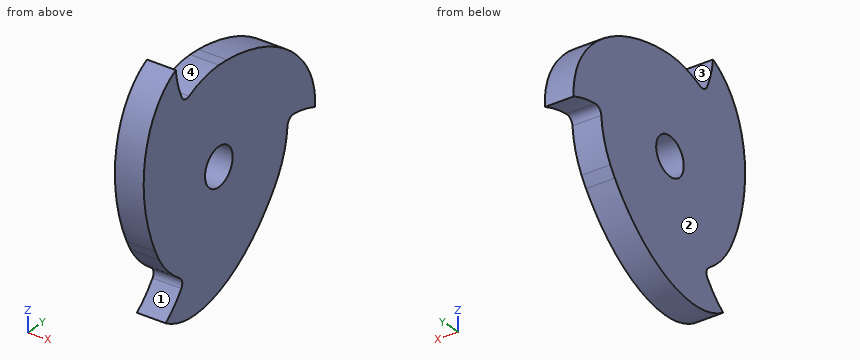
from build123d import *

# Parameters (mm, degrees)
SKETCH1_R           = 6.35
BOSS_EXTRUDE3_DEPTH = 9.525
FILLET3_R           = 2.54


with BuildPart() as part:
    # Sketch1 → Boss-Extrude3 (new body)
    # profile 1 of 4: a face of its own
    with BuildSketch(Plane(origin=(0, 0, 0), x_dir=(0, 0, -1), z_dir=(1, 0, 0))):
        with BuildLine():
            ThreePointArc((-31.520099492, 3.813899322), (-21.059097755, 23.760827043), (0, 31.75))
            ThreePointArc((0, 31.75), (0.675988504, 38.199887052), (2.67457554, 44.369461859))
            add(Edge.make_bspline(
                [(2.67457554, 44.369461859), (-27.656863026, 46.197830298), (-31.520099492, 3.813899322)],
                knots=[3.141592654, 3.141592654, 3.141592654, 4.660979846, 4.660979846, 4.660979846], degree=2, weights=[1, 0.709776495, 0.966045781]))
        make_face()
    # profile 2 of 4: a face of its own
    with BuildSketch(Plane(origin=(0, 0, 0), x_dir=(0, 0, -1), z_dir=(1, 0, 0))):
        with BuildLine():
            add(Edge.make_bspline(
                [(19.062983446, 25.390257228), (17.50131988, 26.492217898), (15.875, 27.49630657)],
                knots=[1.519387193, 1.519387193, 1.519387193, 1.613788447, 1.613788447, 1.613788447], degree=2, weights=[0.966045781, 0.981968084, 1]))
            ThreePointArc((15.875, 27.49630657), (8.217504682, 30.668144985), (0, 31.75))
            ThreePointArc((0, 31.75), (-21.059097755, 23.760827043), (-31.520099492, 3.813899322))
            add(Edge.make_bspline(
                [(-31.520099492, 3.813899322), (-31.693593642, 1.910478667), (-31.75, 0)],
                knots=[4.660979846, 4.660979846, 4.660979846, 4.7553811, 4.7553811, 4.7553811], degree=2, weights=[0.966045781, 0.981968084, 1]))
            ThreePointArc((-31.75, 0), (-30.668144985, -8.217504682), (-27.49630657, -15.875))
            ThreePointArc((-27.49630657, -15.875), (-10.047930956, -30.118127158), (12.457116045, -29.204156551))
            add(Edge.make_bspline(
                [(12.457116045, -29.204156551), (14.192273762, -28.402696564), (15.875, -27.49630657)],
                knots=[1.519387193, 1.519387193, 1.519387193, 1.613788447, 1.613788447, 1.613788447], degree=2, weights=[0.966045781, 0.981968084, 1]))
            ThreePointArc((15.875, -27.49630657), (22.450640303, -22.450640303), (27.49630657, -15.875))
            ThreePointArc((27.49630657, -15.875), (30.668144985, -8.217504682), (31.75, 0))
            ThreePointArc((31.75, 0), (28.401692066, 14.191771834), (19.062983446, 25.390257228))
        make_face()
        with Locations(Location((0, 0, 0), (0, 0, 180))):
            Circle(SKETCH1_R, mode=Mode.SUBTRACT)
    # profile 3 of 4: a face of its own
    with BuildSketch(Plane(origin=(0, 0, 0), x_dir=(0, 0, -1), z_dir=(1, 0, 0))):
        with BuildLine():
            add(Edge.make_bspline(
                [(37.087793352, -24.500981292), (53.836926151, 0.852630821), (19.062983446, 25.390257228)],
                knots=[0, 0, 0, 1.519387193, 1.519387193, 1.519387193], degree=2, weights=[1, 0.709776495, 0.966045781]))
            ThreePointArc((19.062983446, 25.390257228), (28.401692066, 14.191771834), (31.75, 0))
            ThreePointArc((31.75, 0), (30.668144985, -8.217504682), (27.49630657, -15.875))
            ThreePointArc((27.49630657, -15.875), (32.744078357, -19.685366743), (37.087793352, -24.500981292))
        make_face()
    # profile 4 of 4: a face of its own
    with BuildSketch(Plane(origin=(0, 0, 0), x_dir=(0, 0, -1), z_dir=(1, 0, 0))):
        with BuildLine():
            ThreePointArc((-27.49630657, -15.875), (-33.420066861, -18.514520309), (-39.762368892, -19.868480568))
            add(Edge.make_bspline(
                [(-39.762368892, -19.868480568), (-26.180063124, -47.050461119), (12.457116045, -29.204156551)],
                knots=[0, 0, 0, 1.519387193, 1.519387193, 1.519387193], degree=2, weights=[1, 0.709776495, 0.966045781]))
            ThreePointArc((12.457116045, -29.204156551), (-10.047930956, -30.118127158), (-27.49630657, -15.875))
        make_face()
    extrude(amount=BOSS_EXTRUDE3_DEPTH)

    # Fillet3
    fillet3_edges = [part.edges().sort_by_distance(p)[0] for p in [
        (4.7625, 31.75, 0),
        (4.7625, -15.875, -27.49630657),
        (4.7625, -15.875, 27.49630657),
    ]]
    fillet(fillet3_edges, radius=FILLET3_R)


solid = part.part
Work out the finished part from the listing and answer in its coordinate system (mm). Face numbers are marked on the shaded views. Round coordinates to 2 decimals unless told otherwise and drop trailing zeros. One line per question, with ' | ' between items. Start each with the question number.
(1) Flat-ended cylindrical pins translate along their axes: pin 1 Ø1.5 at (x, y) = (3, 5) entering from -Z; pin 2 Ø4 at (x, z) = (4.5, -4) entering from -Y; pin 3 Ø1 at (x, y) = (3.5, 7) entering from -Z. Find the tip coordinate at first contact, or state that the pin passes through.
(2) Find the intervals of material crossed by line 1 (Y direction, x = 6.5, z = -5.5); line 2 (Y direction, x = 6, z = 0); line 3 (Z direction, x = 1, y = -21), in increasing order.
(3) For a pull along Y with two mould halves and no side action, classify the marked faces 1, 2, 3 and 4 as released by +Y, released by -Y, zero draft, split by the parting line, or undercut.
Geometry check:
1) pin 1: stops at z = -37.37 | pin 2: stops at y = -32.93 | pin 3: stops at z = -36.23
2) line 1: y = -31.92 to -3.17, 3.17 to 31.27 | line 2: y = -33.4 to -6.35, 6.35 to 44.37 | line 3: z = -38.98 to -34.12, -23.81 to 39.16
3) face 1: released by -Y | face 2: zero draft | face 3: undercut | face 4: undercut
